Can you work these out from the model? Positions are in its coordinate system, mm. A direction names the side the tool comes from. Give positions to 0.01 mm unless a question says otherwise; leave off trailing zeros. Write each loop counter-clockwise with the first axis right and the second up, starting at its lowest first coordinate (ties: lowest second). Pieces come first, ordered by that corner, then holes.
```python
from build123d import *

# Parameters (mm, degrees)
F0_W     = 423.8752
F0_H     = 69.85
F0_R     = 6.35
F1_DEPTH = 1.397
F2_W     = 423.8752
F2_H     = 11.1125
F3_DEPTH = 1.397
F4_W     = 1.397
F4_H     = 63.754
F5_DEPTH = 12.7


with BuildPart() as f1:
    # F0 (on Front) → F1 (new body)
    with BuildSketch(Plane.XZ):
        Rectangle(F0_W, F0_H)
        with BuildLine():
            ThreePointArc((-130.702728, -29.886292), (-130.702728, -20.906036), (-121.722472, -20.906036))
            Line((-121.722472, -20.906036), (-121.718636, -20.909872))
            ThreePointArc((-121.718636, -20.909872), (-121.718636, -29.890128), (-130.698892, -29.890128))
            Line((-130.698892, -29.890128), (-130.702728, -29.886292))
        make_face(mode=Mode.SUBTRACT)
        with BuildLine():
            ThreePointArc((-130.702728, -4.490128), (-130.702728, 4.490128), (-121.722472, 4.490128))
            Line((-121.722472, 4.490128), (-96.322472, -20.909872))
            ThreePointArc((-96.322472, -20.909872), (-96.322472, -29.890128), (-105.302728, -29.890128))
            Line((-105.302728, -29.890128), (-130.702728, -4.490128))
        make_face(mode=Mode.SUBTRACT)
        with BuildLine():
            ThreePointArc((-96.322472, 4.490128), (-96.322472, -4.490128), (-105.302728, -4.490128))
            Line((-105.302728, -4.490128), (-130.702728, 20.909872))
            ThreePointArc((-130.702728, 20.909872), (-130.702728, 29.890128), (-121.722472, 29.890128))
            Line((-121.722472, 29.890128), (-96.322472, 4.490128))
        make_face(mode=Mode.SUBTRACT)
        with Locations((-100.8126, 25.4)):
            Circle(F0_R, mode=Mode.SUBTRACT)
    extrude(amount=F1_DEPTH)

    # F2 (on face) → F3 (join)
    with BuildSketch(Plane(origin=(0, 0, 0), x_dir=(-1, 0, 0), z_dir=(0, 1, 0))):
        with Locations((0, 38.89375)):
            Rectangle(F2_W, F2_H)
        with Locations((0, -38.89375)):
            Rectangle(F2_W, F2_H)
    extrude(amount=F3_DEPTH)

    # F4 (on face) → F5 (join)
    with BuildSketch(Plane.XZ.offset(1.397)):
        with Locations((-211.9376, 0)):
            Rectangle(F4_W, F4_H)
        with Locations((211.9376, 0)):
            Rectangle(F4_W, F4_H)
    extrude(amount=-F5_DEPTH)


solid = f1.part
```
1) Suppose I cut it at C-C on x = -115. State how many separate pieces and enclosed holes the cut face has, plus the area to 3 significant figures.
Values follow:
separate pieces: 3
enclosed holes: 0
area: 78.4 mm2
2) Suppose I cut it at B-B on z = 0. Write out the boundary of the cut face in (x, y), plus the area to 3 significant figures.
Values follow:
outline: (-212.64, -1.4) - (-132.56, -1.4) - (-132.56, 0) - (-211.24, 0) - (-211.24, 11.3) - (-212.64, 11.3) - close; (-117.23, -1.4) - (-109.79, -1.4) - (-109.79, 0) - (-117.23, 0) - close; (-94.46, -1.4) - (212.64, -1.4) - (212.64, 11.3) - (211.24, 11.3) - (211.24, 0) - (-94.46, 0) - close
area: 583 mm2
3) Suppose I cut it at A-A on y = 4.5. Write out the boundary of the cut face in (x, z).
Values follow:
outline: (-212.64, -31.88) - (-211.24, -31.88) - (-211.24, 31.88) - (-212.64, 31.88) - close; (211.24, -31.88) - (212.64, -31.88) - (212.64, 31.88) - (211.24, 31.88) - close
4) Please list where these lines run through material, in increasing order: L1, parallel to X at y = 3.5, z = -18.5; L2, parallel to X at y = -0.5, z = -2; L3, parallel to Y at x = 88.5, z = -20.
Values follow:
L1: x = -212.64 to -211.24, 211.24 to 212.64
L2: x = -212.64 to -132.24, -115.23 to -107.79, -94.79 to 212.64
L3: y = -1.4 to 0
5) For pin 1 Ø5 at (x, z) = (-17, -29) entering from +Y; pin 2 Ø3 at (x, z) = (-57.5, -42) entering from -Y; pin 3 Ø1.4 at (y, z) = (0.5, 36) entering from -X; pin 4 Ø6 at (x, y) = (83.5, 7) entering from +Z, each with a flat end and sliding along its axis, tell me the tip position at first contact or that it passes through.
Values follow:
pin 1: stops at y = 0
pin 2: stops at y = 0
pin 3: stops at x = -211.94
pin 4: passes through
6) For faces 1 (the face through (3, 0, -40)), 2 (the face through (-212.636, 5, 0)), 3 (the face through (3, 0, 40)), 4 (the face through (-109.2, -0.69, -8.03)), 5 (the face through (3, 1.397, 39)), which set-ups out of +Z, -Z, +X, -X, +Y, -Y let a thin tool reach every point of the face, with its end or its side?
Values follow:
face 1: -Z, +X, -X, -Y
face 2: +Z, -Z, -X, +Y, -Y
face 3: +Z, +X, -X, -Y
face 4: +Y, -Y
face 5: +Z, -Z, +X, -X, +Y
